Geometry: see drawing. Coordinates: mm, zero at the bounding-box minimum. A direction names the side the tool comes from. Give positions to 0.01 mm unless a question says otherwise; leave off trailing zeros. Loops run counter-clockwise (first coordinate to the right, second up) from the corner with the lowest first, then second, coordinate; pieces in that order, holes last. Notation, with made-up numbers: (53.5, 36) -> (83.5, 36) arc R25 ccw to (83.5, 56) -> close; hole circle Ø5 at (-38.5, 40.5). An arc over 180 degrees is marked (long way). One line per question, with ' | ' between items.
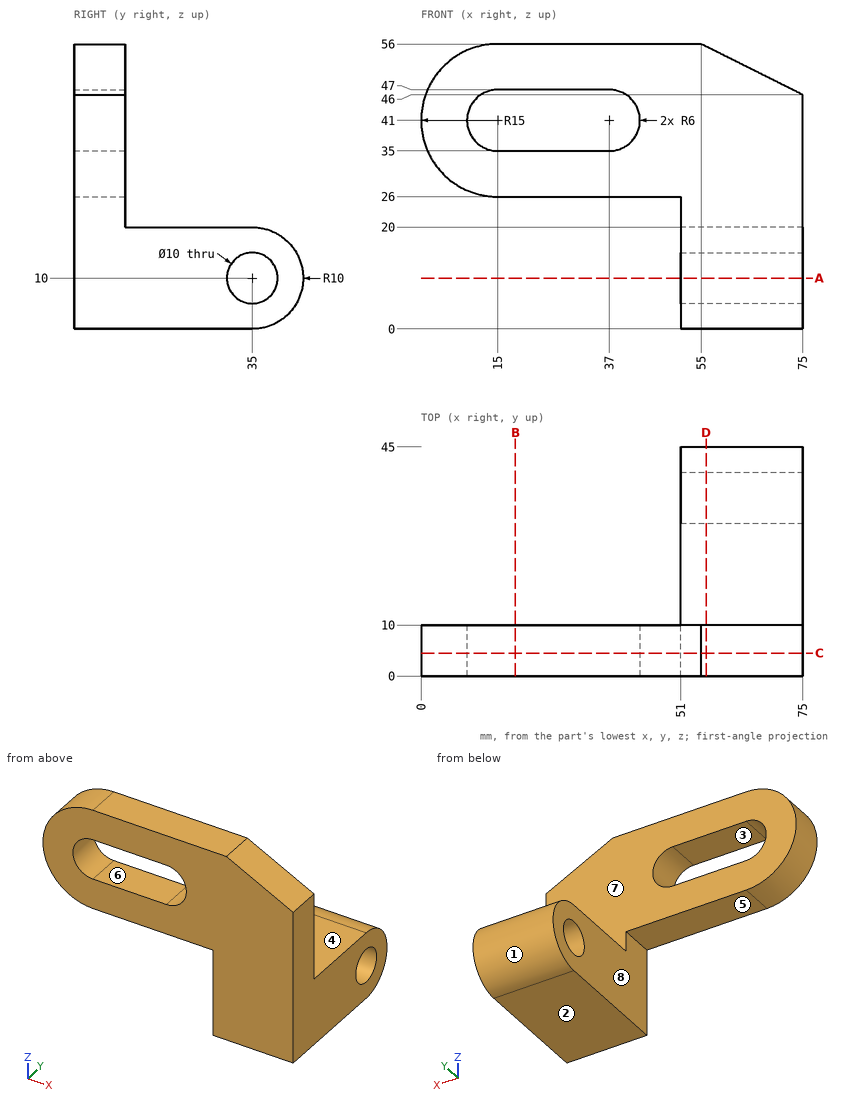
1. Reachability of the marked faces 1, 2, 3, 4 and 5 from +Z, -Z, +X, -X, +Y, -Y: full face, straight path, thin tool, end or side. Return the list, or none.
Determined:
face 1: +X, -X, +Y | face 2: -Z, +X, -X, +Y, -Y | face 3: +Y, -Y | face 4: +Z, +X, -X, +Y | face 5: -Z, -X, +Y, -Y
2. Section query A-A (z = 10). Output: boundary loops of the cut face in (x, y).
Determined:
outline: (51, 0) -> (75, 0) -> (75, 30) -> (51, 30) -> close; (51, 40) -> (75, 40) -> (75, 45) -> (51, 45) -> close
3. Pin query (flat end, axial travel): P1, Ø12, axis at x = 26.5, y = 10.5, coming from the -Z side; P2, Ø8, axis at y = 29.5, z = 9, coming from the -X side; P3, Ø19, axis at x = 58, y = 20, coming from the +Z side. Return the tip coordinate at first contact, or that it passes through.
Determined:
P1: stops at z = 26 | P2: stops at x = 51 | P3: stops at z = 20
4. Section query D-D (x = 56). Output: boundary loops of the cut face in (y, z), then the cut area to 3 significant figures.
Determined:
outline: (0, 0) -> (35, 0) arc R10 ccw to (35, 20) -> (10, 20) -> (10, 55.5) -> (0, 55.5) -> close; hole circle Ø10 at (35, 10) | area: 1,130 mm2
5. Section query B-B (x = 18.5). Output: boundary loops of the cut face in (y, z).
Determined:
outline: (0, 26) -> (10, 26) -> (10, 35) -> (0, 35) -> close; (0, 47) -> (10, 47) -> (10, 56) -> (0, 56) -> close
6. Section query C-C (y = 4.5). Output: boundary loops of the cut face in (x, z), then the cut area to 3 significant figures.
Determined:
outline: (15, 26) -> (51, 26) -> (51, 0) -> (75, 0) -> (75, 46) -> (55, 56) -> (15, 56) arc R15 ccw to start; hole (15, 35) -> (37, 35) arc R6 ccw to (37, 47) -> (15, 47) arc R6 ccw to start | area: 2,300 mm2
7. Pull-direction query (X, two-part tool) for the marked faces 6, 7 and 8; classes: pulls with the +X half, pulls with the -X half, needs draft (parallel to the pull), parting line crosses it, or undercut.
Determined:
face 6: undercut | face 7: needs draft | face 8: pulls with the -X half
8. Ray query, line 1 along Y through (x, z) = (62, 10); line 2 along Z through (x, y) = (25, 4.5); line 3 along X through (y, z) = (40.5, 12.5). Return the intervals inside material, ascending. Write a range as from..to.
Determined:
line 1: y = 0..30, 40..45 | line 2: z = 26..35, 47..56 | line 3: x = 51..75
